CAD build for the part. Positions are in the model's coordinates, mm. Face numbers are marked on the shaded views. Round coordinates to 2 decimals unless told otherwise and drop trailing zeros. Write each loop counter-clockwise with the first axis right and the second up, starting at its lowest first coordinate (ties: lowest second). Pieces come first, ordered by that corner, then holes. Notation, with made-up numbers: (51.5, 67) - (55.5, 67) arc R13 ccw to (55.5, 92) - close; hole circle Ø2 at (81, 12). An arc over 180 degrees is marked (long way). Use one line per item in the form item = value. Start each with the question number.
Item 1: Drill centre lines: L1, parallel to Y at x = 0, z = 56; L2, parallel to X at y = -0.5, z = 68; L3, parallel to Y at x = -7, z = 25. Where is each one in solid material? Low to high.
Item 2: Band-saw the part on C-C, the plane z = 71.5. List the corners of the cut face in (x, y).
Item 3: Pull direction Y, two halves, no side cores. Call the marked faces 1, 2, 3 and 4: +Y half, -Y half, draft (parallel to the pull), parting line (faces both ways), or undercut.
Item 4: Band-saw the part on A-A, the plane x = 0. List the corners of the cut face in (y, z), and give its area (3 significant figures).
Item 5: Pin check, flat tip, straight feed: pin 1 (12 mm diameter, centred on x = 0, y = 0, fed in from +Z). Stop position of the tip, or through.
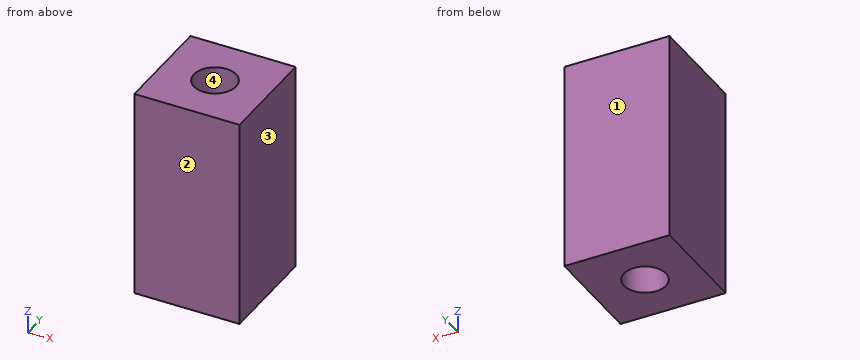
Autodesk Inventor part; units mm, degrees
ref_plane "YZ Plane" through (0, 0, 0) normal (1, 0, 0) x (0, 1, 0)
ref_plane "XZ Plane" through (0, 0, 0) normal (0, 1, 0) x (-1, 0, 0)
ref_plane "XY Plane" through (0, 0, 0) normal (0, 0, 1) x (1, 0, 0)
sketch "Sketch1" plane through (0, 0, 0) normal (0, 0, 1) x (1, 0, 0)
  line L0 (19.05, -19.05) -> (-19.05, -19.05)
  line L1 (-19.05, -19.05) -> (-19.05, 19.05)
  line L2 (-19.05, 19.05) -> (19.05, 19.05)
  line L3 (19.05, 19.05) -> (19.05, -19.05)
  circle A0 centre (0, 0) radius 7.62
  dimension "d0" = 38.1
  dimension "d1" = 15.24
extrude "Extrusion1" add sketch "Sketch1" along normal blind 76.2
properties part number "middleAXIS"
Determined:
q1.L1 = -19.05 to -7.62, 7.62 to 19.05
q1.L2 = -19.05 to -7.6, 7.6 to 19.05
q1.L3 = -19.05 to -3.01, 3.01 to 19.05
q2.outline = (-19.05, -19.05) - (19.05, -19.05) - (19.05, 19.05) - (-19.05, 19.05) - close; hole circle Ø15.24 at (0, 0)
q3.face_1 = +Y half
q3.face_2 = -Y half
q3.face_3 = draft
q3.face_4 = undercut
q4.outline = (-19.05, 0) - (-7.62, 0) - (-7.62, 76.2) - (-19.05, 76.2) - close; (7.62, 0) - (19.05, 0) - (19.05, 76.2) - (7.62, 76.2) - close
q4.area = 1,740 mm²
q5.pin_1 = through
